Could you check a few things on this drawing? It's one solid part, dimensions in mm from its lowest x, y, z. A direction names the side the tool comes from. Round coordinates to 2 decimals unless told otherwise and drop trailing zeros. Order: outer loops, then holes, each group sorted by start corner. A loop starts at its lowest first (then second) coordinate and runs counter-clockwise, first axis right, second up. Notation, with made-up numbers: (77, 76.25) -> (110, 76.25) arc R19 cw to (110, 104.25) -> close; hole circle Ø2 at (9.5, -14.75). An arc over 180 degrees is marked (long way). Use a Markdown table: item, result. Add a question column.
(1) I want a section at D-D, the plane y = 28. Please give me the cut outline in (x, z) (1 decimal), then the cut area to 3 significant figures.
(2) Thinking about a two-plate mould opening in X: for the marked faces 1 and 2, which applies, pulls with the +X half, pulls with the -X half, needs draft (parallel to the pull), parting line crosses it, or undercut?
(3) I want a section at B-B, the plane y = 40. Please give me the cut outline in (x, z) (1 decimal).
(4) I want a section at C-C, the plane x = 57.5. Please give me the cut outline in (y, z) (1 decimal).
(5) I want a section at A-A, the plane z = 4.5. Please give me the cut outline in (x, y).
(6) I'm going to push flat-ended pins straight in: P1, Ø4, axis at x = 20.5, z = 2.5, coming from the -Y side; P2, Ø4, axis at x = 20.5, z = 13, coming from the +Y side; P3, Ø3, axis at y = 43.5, z = 14, coming from the -X side. Where does each tip first touch, or does it pass through?
(7) On a 3-axis mill with a long thin cutter (end or side, diameter ignored), from which of +Z, -Z, +X, -X, +Y, -Y can I reach the whole of each face in a straight line? I mean the marked faces 3 and 4. Say none if no direction works.
(8) If I drill on probe 1 along Z at (x, y) = (20.5, 21.5); probe 2 along X at (y, z) = (50, 3); probe 3 along X at (y, z) = (61.5, 5.75) (1 decimal), over which ranges is the centre line in solid material (lowest first)?
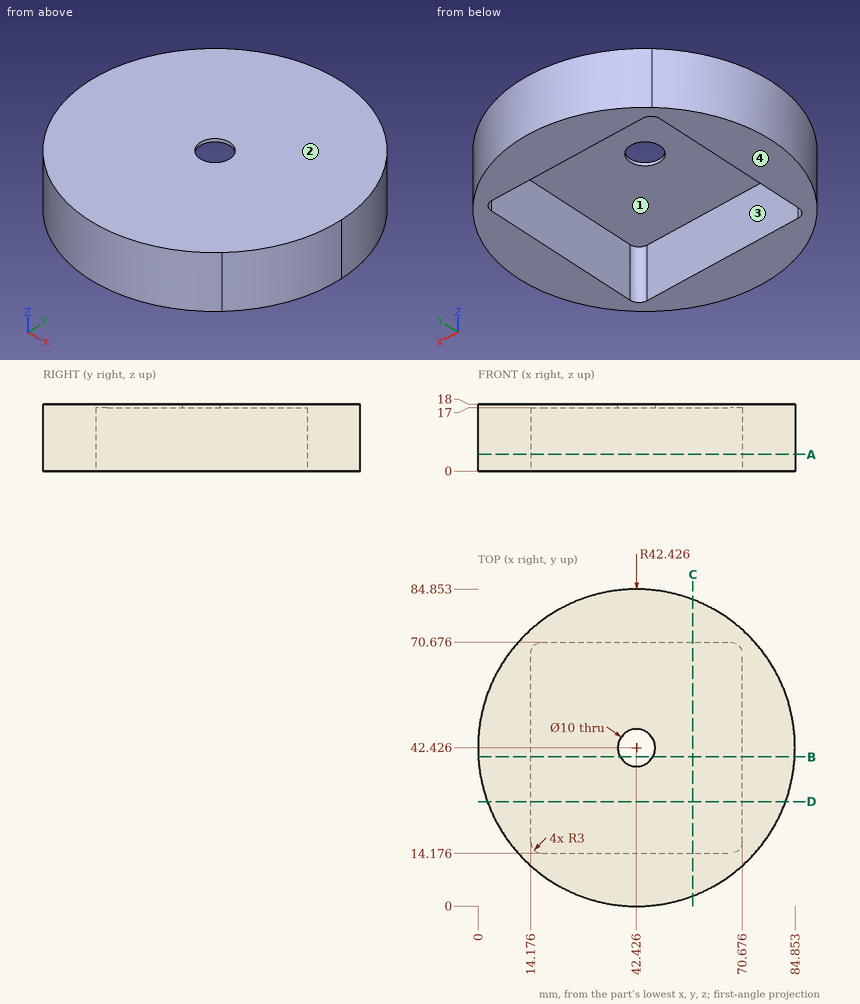
Taken from the geometry:
| question | item | result |
|---|---|---|
| 1 | outline | (2.5, 0) -> (14.2, 0) -> (14.2, 17) -> (70.7, 17) -> (70.7, 0) -> (82.3, 0) -> (82.3, 18) -> (2.5, 18) -> close |
| 1 | area | 476 mm2 |
| 2 | face 1 | undercut |
| 2 | face 2 | needs draft |
| 3 | outline | (0.1, 0) -> (14.2, 0) -> (14.2, 17) -> (38.1, 17) -> (38.1, 18) -> (0.1, 18) -> close; (46.8, 17) -> (70.7, 17) -> (70.7, 0) -> (84.8, 0) -> (84.8, 18) -> (46.8, 18) -> close |
| 4 | outline | (2.8, 0) -> (14.2, 0) -> (14.2, 17) -> (70.7, 17) -> (70.7, 0) -> (82.1, 0) -> (82.1, 18) -> (2.8, 18) -> close |
| 5 | outline | circle Ø84.85 at (42.43, 42.43); hole (14.18, 17.18) arc R3 ccw to (17.18, 14.18) -> (67.68, 14.18) arc R3 ccw to (70.68, 17.18) -> (70.68, 67.68) arc R3 ccw to (67.68, 70.68) -> (17.18, 70.68) arc R3 ccw to (14.18, 67.68) -> close |
| 6 | P1 | stops at y = 4.97 |
| 6 | P2 | stops at y = 79.88 |
| 6 | P3 | stops at x = 0 |
| 7 | face 3 | -Z |
| 7 | face 4 | -Z, +X, -X, +Y, -Y |
| 8 | probe 1 | z = 17 to 18 |
| 8 | probe 2 | x = 0.68 to 14.18, 70.68 to 84.17 |
| 8 | probe 3 | x = 4.5 to 14.2, 70.7 to 80.3 |
